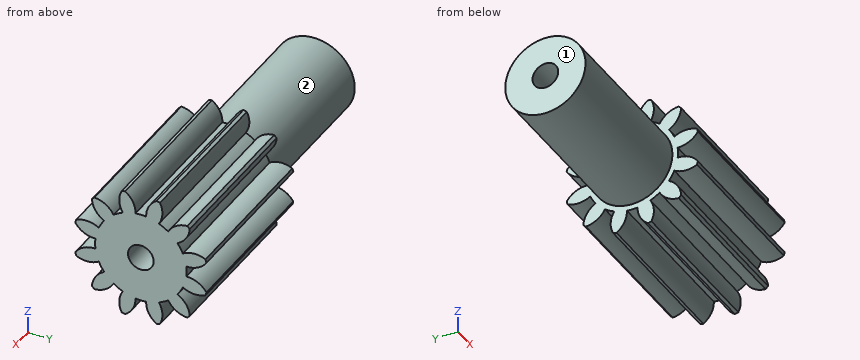
```python
from build123d import *

# Parameters (mm, degrees)
BASPROSKE_W      = 5
BASPROSKE_H      = 2.1
TOOTHCUT_DEPTH   = 6.815496539
TEETHCUTS_COUNT  = 12
TEETHCUTS_ANGLE  = 330
HUBNEAONESKE_R   = 1.25
HUBNEARONE_DEPTH = 5.0000508
BORSKE_R         = 0.4
BORE_DEPTH       = 10.0000508


with BuildPart() as part:
    # BasProSke → Base-Revolve (revolve)
    with BuildSketch(Plane(origin=(0, 0, 0), x_dir=(1, 0, 0), z_dir=(0, 1, 0)), mode=Mode.PRIVATE) as base_revolve_sk:
        with Locations((2.5, 1.05)):
            Rectangle(BASPROSKE_W, BASPROSKE_H)
    revolve(base_revolve_sk.sketch.rotate(Axis((-10, 0, 0), (1, 0, 0)), 180), axis=Axis((-10, 0, 0), (1, 0, 0)))

    # TooCutSke → ToothCut (cut, through all)
    with BuildSketch(Plane(origin=(0, 0, 0), x_dir=(0, 0, -1), z_dir=(1, 0, 0))):
        with BuildLine():
            ThreePointArc((0.16674814, 1.41420333), (0, 1.424), (-0.16674814, 1.41420333))
            ThreePointArc((-0.16674814, 1.41420333), (-0.254548019, 1.786124318), (-0.520302512, 2.060730564))
            ThreePointArc((-0.520302512, 2.060730564), (0, 2.1254), (0.520302512, 2.060730564))
            ThreePointArc((0.520302512, 2.060730564), (0.254548019, 1.786124318), (0.16674814, 1.41420333))
        make_face()
    toothcut = extrude(amount=TOOTHCUT_DEPTH, mode=Mode.SUBTRACT)

    # TeethCuts: ToothCut ×12 about axis
    teethcuts_axis = Axis((-10, 0, 0), (1, 0, 0))
    for i in range(1, TEETHCUTS_COUNT):
        add(toothcut.rotate(teethcuts_axis, i * TEETHCUTS_ANGLE / (TEETHCUTS_COUNT - 1)), mode=Mode.SUBTRACT)

    # HubNeaOneSke → HubNearOne (add)
    with BuildSketch(Plane.ZY):
        with Locations(Location((0, 0, 0), (0, 0, 180))):
            Circle(HUBNEAONESKE_R)
    extrude(amount=HUBNEARONE_DEPTH)

    # BorSke → Bore (cut, symmetric)
    with BuildSketch(Plane(origin=(0, 0, 0), x_dir=(0, 0, -1), z_dir=(1, 0, 0))):
        with Locations(Location((0, 0, 0), (0, 0, 180))):
            Circle(BORSKE_R)
    extrude(amount=BORE_DEPTH, both=True, mode=Mode.SUBTRACT)


solid = part.part
```
CAD build for the part. Positions are in the model's coordinates, mm. Face numbers are marked on the shaded views. A direction names the side the tool comes from. Round coordinates to 2 decimals unless told otherwise and drop trailing zeros. Loops run counter-clockwise (first coordinate to the right, second up) from the corner with the lowest first, then second, coordinate; pieces in that order, holes last. Notation, with made-up numbers: M 46,87 L 78,87 A33 ccw 78,124 Z; hole C -32,76.25 d10. An arc over 180 degrees is marked long. Use a Markdown table: item, result. Add a question column.
(1) Drill centre lines: line 1 (Y direction, x = -0.25, z = 0); line 2 (Y direction, x = 2.5, z = -1.25); line 3 (Z direction, x = -2, y = 1.1). Where is each one in solid material? Low to high.
(2) Flat gauge pin, fed straight in: pin 1 (2 mm diameter, centred on x = 3, z = 1, fed in from -Y). Where does the tip first touch, or does it go through?
(3) Cut at D-D (z = -1.8). Give the cut face in (x, y), and give its area (3 significant figures).
(4) Cut at A-A (y = 0). Give the cut face in (x, z).
(5) Which spindle directions (+Z, -Z, +X, -X, +Y, -Y) get a long thin tool onto all of the face, cutting with end or side? Do the marked faces 1 and 2. Say none if no direction does.
(6) Cut at C-C (x = -1.5). Give the cut face in (y, z).
Geometry says:
| question | item | result |
|---|---|---|
| 1 | line 1 | y = -1.25 to -0.4, 0.4 to 1.25 |
| 1 | line 2 | y = -1.48 to -0.92, -0.68 to 0.68, 0.92 to 1.48 |
| 1 | line 3 | z = -0.59 to 0.59 |
| 2 | pin 1 | stops at y = -2.04 |
| 3 | outline | M 0,-0.66 L 5,-0.66 L 5,-0.26 L 0,-0.26 Z; M 0,0.26 L 5,0.26 L 5,0.66 L 0,0.66 Z |
| 3 | area | 4.02 mm² |
| 4 | outline | M -5,-1.25 L 0,-1.25 L 0,-1.42 L 5,-1.42 L 5,-0.4 L -5,-0.4 Z; M -5,0.4 L 5,0.4 L 5,1.42 L 0,1.42 L 0,1.25 L -5,1.25 Z |
| 5 | face 1 | +Z, -Z, -X, +Y, -Y |
| 5 | face 2 | -X |
| 6 | outline | C 0,0 d2.5; hole C 0,0 d0.8 |
